Here's how the part is built. I have some questions about the finished solid (model axes, mm). Face numbers are marked on the shaded views. A direction names the side the tool comes from. Give positions to 0.01 mm unless a question says otherwise; leave off trailing zeros. Loops run counter-clockwise (first coordinate to the right, second up) from the corner with the lowest first, then second, coordinate; pieces in that order, holes last.
Q1. If we section it at C-C (y = 0): Please give me the cut outline in (x, z), plus the area to 3 significant figures.
Q2. For the marked faces 3, 4 and 5, which set-ups out of +Z, -Z, +X, -X, +Y, -Y let a thin tool reach every point of the face, with its end or its side?
Q3. If we section it at A-A (x = 32): Please give me the cut outline in (y, z).
Q4. If we section it at B-B (y = -12): Please give me the cut outline in (x, z), plus the area to 3 significant figures.
Q5. We'd pull the mould along X, two halves only. Please class the marked faces 1 and 2: +X half, -X half, draft (parallel to the pull), parting line (faces both ways), or undercut.
Q6. I need wall thicknesses on line 1 (Y direction, x = 0, z = 1.05); line 2 (X direction, y = 80, z = -0.8); line 3 (Z direction, x = 18.5, y = 26). Which ranges of each line are inside material? Lowest first, please.
Q7. Will these pins go through, and if not, where does the flat tip stop? P1, Ø6.5, axis at x = 33, y = -9.5, coming from the +Z side; P2, Ø0.6, axis at x = 51.5, z = 1, coming from the -Y side; P3, Ø2.5, axis at x = 12, z = -3, coming from the +Y side.
Q8. If we section it at D-D (x = 56): Please give me the cut outline in (y, z), plus the area to 3 significant figures.
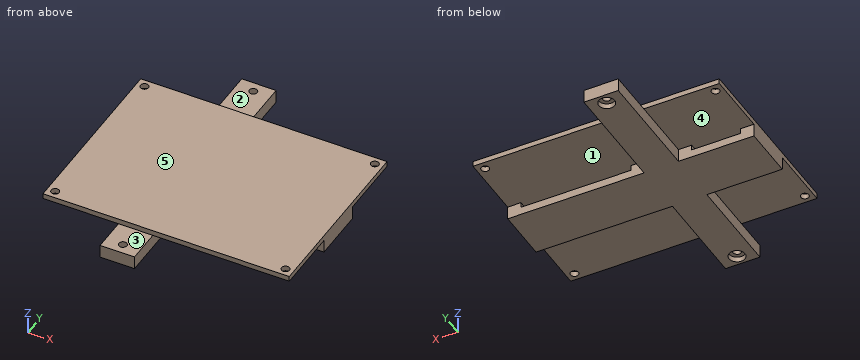
Autodesk Inventor part; units mm, degrees
ref_plane "YZ Plane" through (0, 0, 0) normal (1, 0, 0) x (0, 1, 0)
ref_plane "XZ Plane" through (0, 0, 0) normal (0, 1, 0) x (-1, 0, 0)
ref_plane "XY Plane" through (0, 0, 0) normal (0, 0, 1) x (1, 0, 0)
sketch "Boceto1" plane through (0, 0, 0) normal (0, 0, 1) x (1, 0, 0)
  line L0 (0, 0) -> (87, 0)
  line L1 (87, 63) -> (0, 63)
  circle A0 centre (0, 63) radius 1.5
  circle A1 centre (87, 63) radius 1.5
  circle A2 centre (87, 0) radius 1.5
  circle A3 centre (0, 0) radius 1.5
  line L2 (0, -3) -> (87, -3)
  line L3 (87, -3) -> (90, -3)
  line L4 (90, -3) -> (90, 63)
  line L5 (90, 63) -> (90, 66)
  line L6 (90, 66) -> (0, 66)
  line L7 (0, 66) -> (-3, 66)
  line L8 (-3, 66) -> (-3, -3)
  line L9 (-3, -3) -> (0, -3)
  dimension "d0" = 87
  dimension "d1" = 63
  dimension "d2" = 3
  dimension "d3" = 3
  dimension "d4" = 3
  dimension "d5" = 3
  dimension "d8" = 3
  dimension "d9" = 3
  dimension "d10" = 3
extrude "Extrusión1" add sketch "Boceto1" along normal blind 2
sketch "Boceto2" plane through (0, 0, 0) normal (0, 0, -1) x (-1, 0, 0)
  line L0 (0, 0) -> (0, -12)
  circle A0 centre (0, 63) radius 1.5
  line L1 (0, 63) -> (0, 80)
  line L2 (0, 80) -> (-32, 80)
  line L3 (0, -12) -> (-32, -12)
  circle A1 centre (-32, 80) radius 1.5
  circle A2 centre (-32, -12) radius 1.5
  line L4 (-32, 80) -> (-25.5, 80)
  line L5 (-25.5, 80) -> (-25.5, 84)
  line L6 (-25.5, 84) -> (-38.5, 84)
  line L7 (-38.5, 84) -> (-38.5, 66)
  line L8 (-90, 66) -> (3, 66)
  line L9 (-25.5, 80) -> (-25.5, 66)
  line L10 (-38.5, -12) -> (-38.5, -2.9941)
  line L11 (-38.5, -12) -> (-38.5, -16)
  line L12 (-38.5, -16) -> (-25.5, -16)
  line L13 (-25.5, -16) -> (-25.5, -3)
  line L14 (3, -3) -> (-90, -3)
  line L15 (3, 66) -> (3, -3)
  line L16 (3, 31.5) -> (3, 41.5)
  line L17 (3, 31.5) -> (3, 21.5)
  line L18 (-90, -3) -> (-90, 66)
  line L19 (-90, 21.5) -> (-90, 41.5)
  line L20 (-90, 41.5) -> (-38.5, 41.5)
  line L21 (-38.5, 41.5) -> (-38.5, 66)
  line L22 (3, 41.5) -> (-25.5, 41.5)
  line L23 (-38.5, -2.9941) -> (-38.5, 21.5)
  line L24 (-25.5, 66) -> (-25.5, 41.5)
  line L25 (-25.5, -3) -> (-25.5, 21.5)
  line L26 (-38.5, 21.5) -> (-90, 21.5)
  line L27 (-25.5, 21.5) -> (3, 21.5)
  dimension "d13" = 12
  dimension "d14" = 17
  dimension "d15" = 32
  dimension "d16" = 3
  dimension "d17" = 3
  dimension "d18" = 6.5
  dimension "d19" = 4
  dimension "d20" = 13
  dimension "d21" = 4
  dimension "d22" = 10
  dimension "d23" = 10
  dimension "d24" = 20
extrude "Extrusión2" add sketch "Boceto2" along normal blind 5 contours L13 L12 L11 L10 L14 | L14 L10 L23 L26 L18 L20 L21 L8 L24 L22 L15 L27 L25 | L8 L7 L6 L5 L9
sketch "Boceto3" plane through (0, 0, -5) normal (0, 0, -1) x (-1, 0, 0)
  circle A0 centre (-32, 80) radius 1.5
  circle A1 centre (-32, 80) radius 3
  circle A2 centre (-32, -12) radius 1.5
  circle A3 centre (-32, -12) radius 3
  point P0 (0, 0)
  dimension "d27" = 6
  dimension "d28" = 6
extrude "Extrusión3" cut sketch "Boceto3" against normal blind 2
sketch "Boceto4" plane through (38.5, 41.5, 0) normal (0, 1, 0) x (1, 0, 0)
  line L0 (51.5, 0) -> (51.5, 5)
  line L1 (51.5, 0) -> (46.5, 0)
  line L2 (51.5, 0) -> (0, 0)
  line L3 (46.5, 0) -> (46.5, 2)
  line L4 (46.5, 2) -> (5, 2)
  line L5 (5, 2) -> (5, 0)
  line L6 (5, 0) -> (46.5, 0)
  line L7 (-41.5, 0) -> (-13, 0)
  line L8 (-13, 0) -> (-18, 0)
  line L9 (-18, 0) -> (-18, 2)
  line L10 (-18, 2) -> (-36.5, 2)
  line L11 (-36.5, 2) -> (-36.5, 0)
  line L12 (-36.5, 0) -> (-18, 0)
  point P0 (-38.5, 0)
  dimension "d31" = 5
  dimension "d32" = 2
  dimension "d33" = 41.5
  dimension "d34" = 5
  dimension "d35" = 18.5
extrude "Extrusión4" cut sketch "Boceto4" against normal up to surface (20 mm away)
properties part number "soporte_odroid_xu3"
Check sheet entries:
1. outline: (-3, 0) - (-1.5, 0) - (-1.5, 2) - (-3, 2) - close; (1.5, 0) - (25.5, 0) - (25.5, -5) - (38.5, -5) - (38.5, 0) - (85.5, 0) - (85.5, 2) - (1.5, 2) - close; (88.5, 0) - (90, 0) - (90, 2) - (88.5, 2) - close
1. area: 239 mm2
2. face 3: +Z, +X, -X, -Y
2. face 4: none
2. face 5: +Z, +X, -X, +Y, -Y
3. outline: (-16, -5) - (-15, -5) - (-15, -3) - (-13.5, -3) - (-13.5, 0) - (-16, 0) - close; (-10.5, -3) - (-9, -3) - (-9, -5) - (77, -5) - (77, -3) - (78.5, -3) - (78.5, 0) - (66, 0) - (66, 2) - (-3, 2) - (-3, 0) - (-10.5, 0) - close; (81.5, -3) - (83, -3) - (83, -5) - (84, -5) - (84, 0) - (81.5, 0) - close
4. outline: (25.5, -5) - (29, -5) - (29, -3) - (30.5, -3) - (30.5, 0) - (25.5, 0) - close; (33.5, -3) - (35, -3) - (35, -5) - (38.5, -5) - (38.5, 0) - (33.5, 0) - close
4. area: 44.0 mm2
5. face 1: undercut
5. face 2: draft
6. line 1: y = -3 to -1.5, 1.5 to 61.5, 64.5 to 66
6. line 2: x = 25.5 to 30.5, 33.5 to 38.5
6. line 3: z = -5 to -2, 0 to 2
7. P1: stops at z = 0
7. P2: stops at y = -3
7. P3: stops at y = 41.5
8. outline: (-3, 0) - (66, 0) - (66, 2) - (-3, 2) - close; (21.5, -5) - (41.5, -5) - (41.5, -2) - (21.5, -2) - close
8. area: 198 mm2
